Verification items for this drawing (mm, ordinates from the low corner). A direction names the side the tool comes from. Coordinates: 2 decimals unless noted, no trailing zeros. Order: outer loops, then holes, each group sorted by start corner. A loop starts at its lowest first (then second) coordinate and runs counter-clockwise, first axis right, second up. Notation, with made-up numbers: (18, 31.25) -> (34, 31.25) arc R25 cw to (34, 51.25) -> close; hole circle Ø3 at (-0.5, -25.75). An arc over 180 degrees is marked (long way). Write each question's results on one line, items separated by ' | '. Start each with the question number.
(1) Cross-section at D-D on z = 281.5. Enter the section's corners in (x, y) (1 decimal).
(2) Cross-section at B-B on z = 41.5. Enter the section's corners in (x, y) (1 decimal), and give its area (3 significant figures).
(3) Go/stop test with flat-tipped pins: pin 1 (24 mm diameter, centred on x = 48, z = 219.5, fed in from +Y); pin 2 (1.5 mm diameter, centred on y = 21.5, z = 63, fed in from -X); pin 3 (17 mm diameter, centred on y = 28, z = 230.5, fed in from -X). Record where each tip stops, or that it passes through.
(4) Thickness scan on probe 1 along Z at (x, y) = (62.5, 51.5); probe 2 along Y at (x, z) = (22, 317.5) (1 decimal); probe 3 along X at (y, z) = (26.5, 312). Record the ranges inside material, lowest first. Write a range as [from, to].
(5) Cross-section at A-A on x = 46.5. Enter the section's corners in (y, z) (1 decimal).
(6) Set-up check for the marked faces 1, 2 and 3: record each of +Z, -Z, +X, -X, +Y, -Y from which the full face is reachable in a straight line by a thin tool's end or side.
(7) Cross-section at C-C on y = 59.5. Enter the section's corners in (x, z).
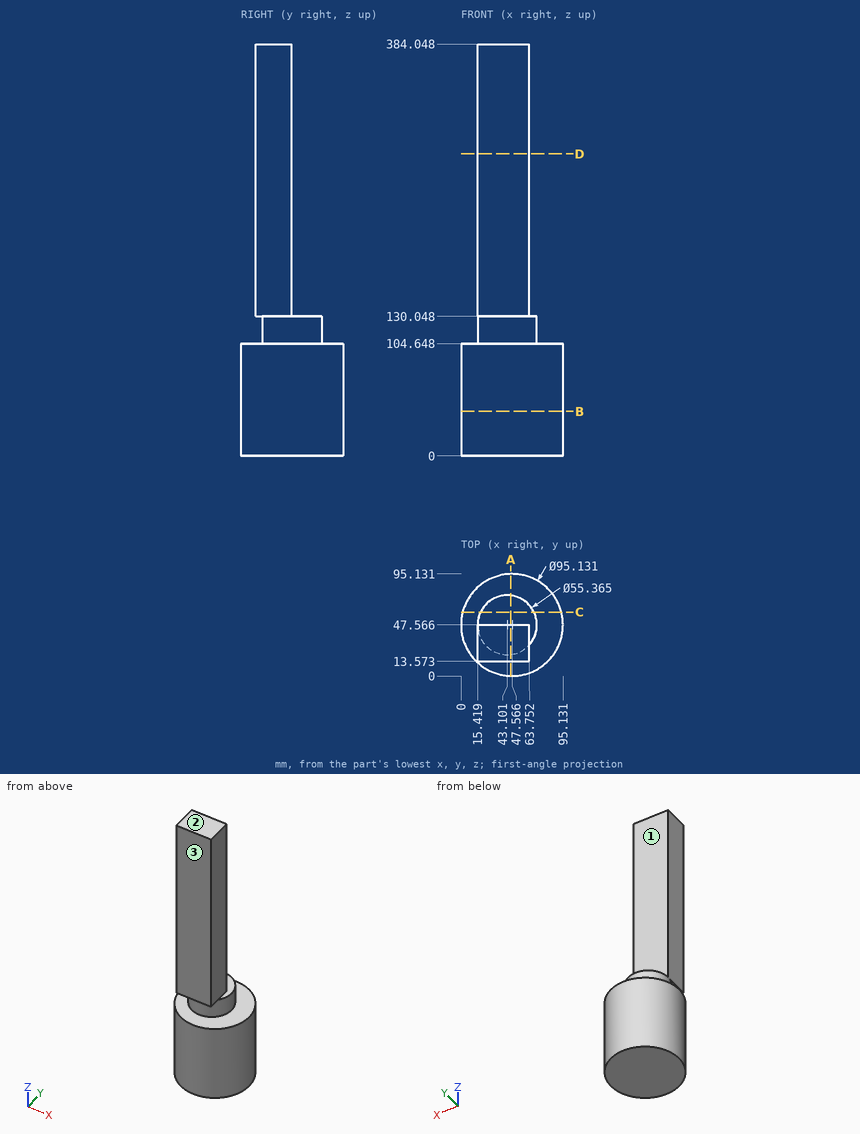
Results are:
1) outline: (15.4, 13.6) -> (63.8, 13.6) -> (63.8, 47.6) -> (15.4, 47.6) -> close
2) outline: circle Ø95.1 at (47.6, 47.6) | area: 7,110 mm2
3) pin 1: stops at y = 47.57 | pin 2: stops at x = 7.3 | pin 3: stops at x = 15.42
4) probe 1: z = [0, 130.05] | probe 2: y = [13.6, 47.6] | probe 3: x = [15.42, 63.75]
5) outline: (0, 0) -> (95.1, 0) -> (95.1, 104.6) -> (75, 104.6) -> (75, 130) -> (47.6, 130) -> (47.6, 384) -> (13.6, 384) -> (13.6, 130) -> (20.1, 130) -> (20.1, 104.6) -> (0, 104.6) -> close
6) face 1: +Z, +X, -X, +Y | face 2: +Z, +X, -X, +Y, -Y | face 3: +Z, +X, -X, -Y
7) outline: (1.52, 0) -> (93.61, 0) -> (93.61, 104.65) -> (68.08, 104.65) -> (68.08, 130.05) -> (18.12, 130.05) -> (18.12, 104.65) -> (1.52, 104.65) -> close
